Geometry: see drawing. Coordinates: mm, zero at the bounding-box minimum. A direction names the side the tool comes from. Coordinates: 2 decimals unless noted, no trailing zeros. Loops run counter-clockwise (first coordinate to the right, second up) from the corner with the lowest first, then second, coordinate; pieces in that order, holes last. Notation, with made-up numbers: (79, 68.5) - (103, 68.5) arc R13 ccw to (103, 76.5) - close; hole circle Ø8 at (8, 28). An arc over 180 degrees is marked (long way). Use one line per item in the form item = value.
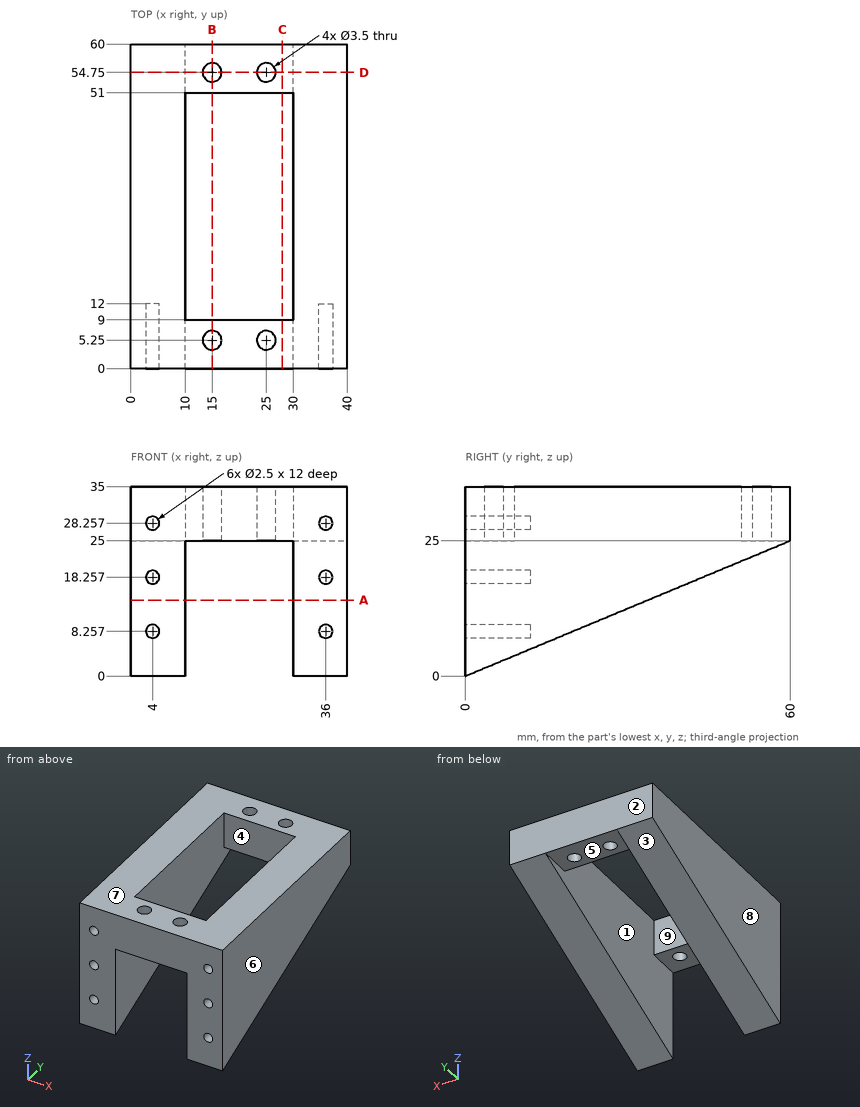
Q1. First-contact query: P1, Ø1.5, axis at y = 7.5, z = 18, coming from the -X side; P2, Ø10, axis at x = 20.5, y = 54.5, coming from the -Z side; P3, Ø1.2, axis at x = 4, z = 18, coming from the -Y side; P4, Ø1.5, axis at x = 4, z = 18.26, coming from the +Y side (1 decimal). Flat tips, straight axial feed; report the tip coordinate or a pass-through.
Check values:
P1 = 0
P2 = 25
P3 = 12
P4 = 45.6
Q2. Pull-direction query (X, two-part tool) for the marked faces 6, 7, 8 and 9; classes: pulls with the +X half, pulls with the -X half, needs draft (parallel to the pull), parting line crosses it, or undercut.
Check values:
face_6 = pulls with the +X half
face_7 = needs draft
face_8 = pulls with the -X half
face_9 = undercut
Q3. Cut plane B-B, the plane x = 15. Return loops of the section in (y, z).
Check values:
outline = (0, 25) - (3.5, 25) - (3.5, 35) - (0, 35) - close; (7, 25) - (9, 25) - (9, 35) - (7, 35) - close; (51, 25) - (53, 25) - (53, 35) - (51, 35) - close; (56.5, 25) - (60, 25) - (60, 35) - (56.5, 35) - close
Q4. Cut plane A-A, the plane z = 14. Return loops of the section in (x, y).
Check values:
outline = (0, 0) - (10, 0) - (10, 33.6) - (0, 33.6) - close; (30, 0) - (40, 0) - (40, 33.6) - (30, 33.6) - close
Q5. Cut plane D-D, the plane y = 54.75. Return loops of the section in (x, z), then the cut area to 3 significant figures.
Check values:
outline = (0, 22.81) - (10, 22.81) - (10, 25) - (13.25, 25) - (13.25, 35) - (0, 35) - close; (16.75, 25) - (23.25, 25) - (23.25, 35) - (16.75, 35) - close; (26.75, 25) - (30, 25) - (30, 22.81) - (40, 22.81) - (40, 35) - (26.75, 35) - close
area = 374 mm²
Q6. Set-up query: the marked faces 1, 2, 3, 4 and 5. Return all of +Z, -Z, +X, -X, +Y, -Y with unobstructed straight access to the full face (end or side cutting, diameter ignored); none if empty.
Check values:
face_1 = -Z
face_2 = +Z, -Z, +X, -X, +Y
face_3 = -Z, +X, -X, +Y
face_4 = +Z, -Z
face_5 = -Z, +Y, -Y
Q7. Cut plane C-C, the plane x = 28. Return loops of the section in (y, z).
Check values:
outline = (0, 25) - (9, 25) - (9, 35) - (0, 35) - close; (51, 25) - (60, 25) - (60, 35) - (51, 35) - close
Q8. Ray query, line 1 along Y through (x, z) = (15, 26); line 2 along Z through (x, y) = (36, 3); line 3 along Y through (x, z) = (21, 27.5). Return the intervals inside material, ascending. Write a range as [from, to].
Check values:
line_1 = [0, 3.5], [7, 9], [51, 53], [56.5, 60]
line_2 = [1.25, 7.01], [9.51, 17.01], [19.51, 27.01], [29.51, 35]
line_3 = [0, 9], [51, 60]
